For this review, take the finished solid that the model builds, in its own axes (mm). Face numbers are marked on the shaded views. Coordinates: 2 decimals unless noted, no trailing zeros. Loops run counter-clockwise (first coordinate to the right, second up) from the corner with the lowest first, then second, coordinate; pieces in that order, holes last. Notation, with made-up numbers: (62.25, 69.25) - (120.25, 69.25) arc R26 cw to (120.25, 106.25) - close; hole circle Ø10 at (46.5, 81.25). An arc over 180 degrees is marked (long way). Answer as a JSON object with one key per item and string values. Group by question number.
Item 1: To check wall thickness, follow line 1 (Y direction, x = 0, z = 0); line 2 (Z direction, x = -11, y = -5.5); line 3 (X direction, y = 11.5, z = -12). State the ranges of each line that lie inside material, in increasing order.
Item 2: Clearance check with flat-ended pins moving along their axes: pin 1 (6 mm diameter, centred on x = 13, z = -32, fed in from -Y); pin 2 (8 mm diameter, centred on x = 2, y = 5, fed in from +Z); pin 3 (6 mm diameter, centred on y = -9.5, z = -1, fed in from +X). State where each tip first meets the part, or that it passes through.
Item 3: We need section C-C (z = -2.5). Give the boundary of the cut face in (x, y).
Item 4: We need section A-A (y = 0). Give the boundary of the cut face in (x, z), then the cut area to 3 significant figures.
Item 5: Mouldability with a two-part tool opening along X and no side actions: class the marked faces 1, 2 and 3 as released by +X, released by -X, zero draft, split by the parting line, or undercut.
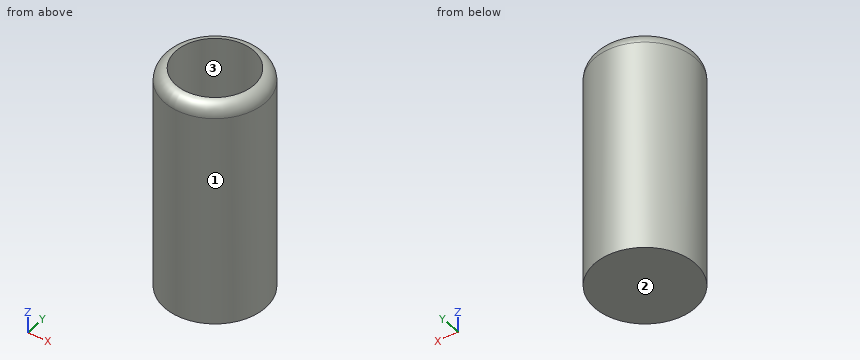
from build123d import *

# Parameters (mm, degrees)
F0_W     = 19.7259690613
F0_H     = 88.3059669286
F2_R     = 15.24
F3_DEPTH = 87.63


# Not quite as in the source:
# - a fillet or chamfer that OpenCascade refuses, or shapes differently, is made with other operations: its cross-section is extruded or revolved along the edge and cut away or added


with BuildPart() as f1:
    # F0 (on Front) → F1 (revolve)
    with BuildSketch(Plane.XZ):
        with Locations((9.8629845306, -15.7623393461)):
            Rectangle(F0_W, F0_H)
    revolve(axis=Axis((0, 0, 0), (0, 0, -1)))

    # F2 (on face) → F3 (cut)
    with BuildSketch(Plane.XY.offset(28.3906441182)):
        Circle(F2_R)
    extrude(amount=-F3_DEPTH, mode=Mode.SUBTRACT)

    # F4: fillet of radius 5.08 on 1 edges, made by hand

    # F4_s1 → F4_t2 (revolve, cut)
    with BuildSketch(Plane.XZ):
        with BuildLine():
            ThreePointArc((15.24, 28.3906441182), (18.4422881448, 26.7210487336), (19.7259690613, 23.345495236))
            Line((19.7259690613, 23.345495236), (19.7259690613, 28.3906441182))
            Line((19.7259690613, 28.3906441182), (15.24, 28.3906441182))
        make_face()
    revolve(axis=Axis((0, 0, 28.3906441182), (0, 0, -1)), mode=Mode.SUBTRACT)


solid = f1.part
Check sheet entries:
{
 "1": {"line 1": "y = -19.73 to -15.24, 15.24 to 19.73", "line 2": "z = -59.92 to -59.24", "line 3": "x = -16.03 to -10, 10 to 16.03"},
 "2": {"pin 1": "stops at y = -17", "pin 2": "stops at z = -59.24", "pin 3": "stops at x = 18.62"},
 "3": {"outline": "circle Ø39.45 at (0, 0); hole circle Ø30.48 at (0, 0)"},
 "4": {"outline": "(-19.73, -59.92) - (19.73, -59.92) - (19.73, 23.35) arc R5.08 ccw to (15.24, 28.39) - (15.24, -59.24) - (-15.24, -59.24) - (-15.24, 28.39) arc R5.08 ccw to (-19.73, 23.35) - close", "area": "802 mm2"},
 "5": {"face 1": "split by the parting line", "face 2": "zero draft", "face 3": "undercut"}
}
